Source: three-view drawing plus pictorial views. Frame: mm from the lowest corner of the part. A direction names the side the tool comes from. Coordinates: 2 decimals unless noted, no trailing zeros. Order: outer loops, then holes, each group sorted by start corner. A loop starts at its lowest first (then second) coordinate and runs counter-clockwise, first axis right, second up. Notation, with made-up numbers: (35.25, 77) - (56.25, 77) arc R14 ccw to (56.25, 100) - close; hole circle Ø1 at (15.5, 16). An arc over 180 degrees is marked (long way). One line per question, with ' | ' between items.
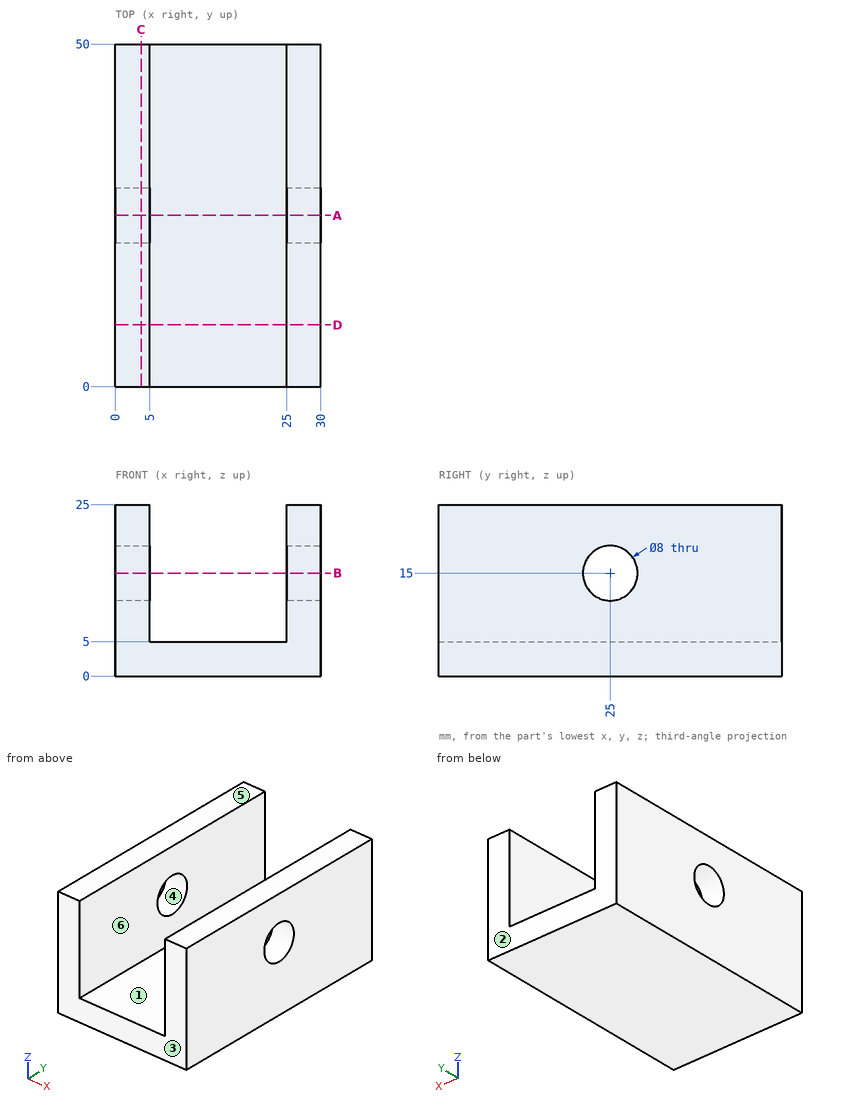
(1) Pin query (flat end, axial travel): P1, Ø5, axis at y = 25, z = 15, coming from the +X side; P2, Ø4, axis at x = 9, z = 4.5, coming from the -Y side; P3, Ø6, axis at x = 18.5, y = 25.5, coming from the +Z side. Return the tip coordinate at first contact, or that it passes through.
Taken from the geometry:
P1: passes through | P2: stops at y = 0 | P3: stops at z = 5
(2) Material intervals for L1, parallel to Y at x = 27, z = 15; L2, parallel to X at y = 32, z = 17; L3, parallel to Z at x = 11.25, y = 17.5, sorted ascending. Write a range as from..to.
Taken from the geometry:
L1: y = 0..21, 29..50 | L2: x = 0..5, 25..30 | L3: z = 0..5
(3) Cut plane A-A (y = 25). Return the cut outline in (x, z).
Taken from the geometry:
outline: (0, 0) - (30, 0) - (30, 11) - (25, 11) - (25, 5) - (5, 5) - (5, 11) - (0, 11) - close; (0, 19) - (5, 19) - (5, 25) - (0, 25) - close; (25, 19) - (30, 19) - (30, 25) - (25, 25) - close
(4) Cut plane B-B (z = 15). Return the cut outline in (x, y).
Taken from the geometry:
outline: (0, 0) - (5, 0) - (5, 21) - (0, 21) - close; (0, 29) - (5, 29) - (5, 50) - (0, 50) - close; (25, 0) - (30, 0) - (30, 21) - (25, 21) - close; (25, 29) - (30, 29) - (30, 50) - (25, 50) - close
(5) Set-up query: the marked faces 5 and 6. Return all of +Z, -Z, +X, -X, +Y, -Y with unobstructed straight access to the full face (end or side cutting, diameter ignored); none if empty.
Taken from the geometry:
face 5: +Z, +X, -X, +Y, -Y | face 6: +Z, +Y, -Y
(6) Cut plane C-C (x = 3.75). Return the cut outline in (y, z), and give its area (3 significant figures).
Taken from the geometry:
outline: (0, 0) - (50, 0) - (50, 25) - (0, 25) - close; hole circle Ø8 at (25, 15) | area: 1,200 mm²
(7) Pull-direction query (Y, two-part tool) for the marked faces 1, 2, 3 and 4; classes: pulls with the +Y half, pulls with the -Y half, needs draft (parallel to the pull), parting line crosses it, or undercut.
Taken from the geometry:
face 1: needs draft | face 2: pulls with the +Y half | face 3: pulls with the -Y half | face 4: undercut
(8) Cut plane D-D (y = 9). Return the cut outline in (x, z).
Taken from the geometry:
outline: (0, 0) - (30, 0) - (30, 25) - (25, 25) - (25, 5) - (5, 5) - (5, 25) - (0, 25) - close
